Geometry check sheet. Reference: the model listing, model coordinates, mm. A direction names the side the tool comes from. Coordinates: 2 decimals unless noted, no trailing zeros. Write each loop counter-clockwise with the first axis right and the second up, starting at its lowest first coordinate (ties: lowest second). Pieces come first, ordered by that corner, then holes.
Autodesk Inventor part; units mm, degrees
ref_plane "YZ Plane" through (0, 0, 0) normal (1, 0, 0) x (0, 1, 0)
ref_plane "XZ Plane" through (0, 0, 0) normal (0, 1, 0) x (-1, 0, 0)
ref_plane "XY Plane" through (0, 0, 0) normal (0, 0, 1) x (1, 0, 0)
sketch "Sketch1" plane through (0, 0, 0) normal (0, 0, 1) x (1, 0, 0)
  line L0 (0, 0) -> (20, 0)
  line L1 (20, 0) -> (20, 3)
  line L2 (0, 3) -> (20, 3)
  line L3 (0, 0) -> (0, 3)
  line L4 (0, -95.4) -> (20, -95.4)
  line L5 (20, -95.4) -> (20, -92.4)
  line L6 (0, -92.4) -> (20, -92.4)
  line L7 (0, -95.4) -> (0, -92.4)
  line L8 (-7.5, 3) -> (0, 3) construction
  line L9 (20, 3) -> (27.5, 3) construction
  line L10 (20, -95.4) -> (27.5, -95.4) construction
  line L11 (-7.5, -95.4) -> (0, -95.4) construction
  line L12 (-7.5, 3) -> (27.5, 3)
  line L13 (27.5, -95.4) -> (-7.5, -95.4)
  line L14 (-7.5, 3) -> (27.5, -95.4) construction
  line L15 (27.5, 3) -> (-7.5, -95.4) construction
  line L16 (-7.5, -95.4) -> (-7.5, -70.567)
  line L17 (-7.5, -21.833) -> (-7.5, 3)
  line L18 (27.5, 3) -> (27.5, -21.833)
  line L19 (27.5, -70.567) -> (27.5, -95.4)
  arc A0 (27.5, -70.567) -> (27.5, -21.833) centre (10, -46.2) ccw
  arc A1 (-7.5, -21.833) -> (-7.5, -70.567) centre (10, -46.2) ccw
  dimension "d1" = 35
  dimension "d2" = 35
extrude "Extrusion1" add sketch "Sketch1" against normal blind 3 contours L0 L1 L12 L18 A0 L19 L13 L5 L6 L7 L16 A1 L17 L3
sketch "Sketch2" plane through (0, 0, -3) normal (0, 0, -1) x (-1, 0, 0)
  arc A0 (0.6, -86.2) -> (4.4, -86.2) centre (2.5, -86.2) ccw construction
  line L0 (0.6, -86.2) -> (0.6, -83.5) construction
  arc A1 (4.4, -83.5) -> (0.6, -83.5) centre (2.5, -83.5) ccw construction
  line L1 (4.4, -83.5) -> (4.4, -86.2) construction
  arc A2 (-1.5, -77.8) -> (-2.5, -78.8) centre (-1.5, -78.8) ccw construction
  line L2 (-2.5, -78.8) -> (-2.5, -91.4) construction
  line L3 (-2.5, -91.4) -> (7.5, -91.4) construction
  line L4 (7.5, -91.4) -> (7.5, -78.8) construction
  arc A3 (7.5, -78.8) -> (6.5, -77.8) centre (6.5, -78.8) ccw construction
  line L5 (6.5, -77.8) -> (-1.5, -77.8) construction
  arc A4 (-24.4, -86.2) -> (-20.6, -86.2) centre (-22.5, -86.2) ccw construction
  line L6 (-24.4, -86.2) -> (-24.4, -83.5) construction
  arc A5 (-20.6, -83.5) -> (-24.4, -83.5) centre (-22.5, -83.5) ccw construction
  line L7 (-20.6, -83.5) -> (-20.6, -86.2) construction
  arc A6 (-26.5, -77.8) -> (-27.5, -78.8) centre (-26.5, -78.8) ccw construction
  line L8 (-27.5, -78.8) -> (-27.5, -91.4) construction
  line L9 (-27.5, -91.4) -> (-17.5, -91.4) construction
  line L10 (-17.5, -91.4) -> (-17.5, -78.8) construction
  arc A7 (-17.5, -78.8) -> (-18.5, -77.8) centre (-18.5, -78.8) ccw construction
  line L11 (-18.5, -77.8) -> (-26.5, -77.8) construction
  arc A8 (4.4, -6.2) -> (0.6, -6.2) centre (2.5, -6.2) ccw construction
  line L12 (4.4, -6.2) -> (4.4, -8.9) construction
  arc A9 (0.6, -8.9) -> (4.4, -8.9) centre (2.5, -8.9) ccw construction
  line L13 (0.6, -8.9) -> (0.6, -6.2) construction
  arc A10 (6.5, -14.6) -> (7.5, -13.6) centre (6.5, -13.6) ccw construction
  line L14 (7.5, -13.6) -> (7.5, -1) construction
  line L15 (7.5, -1) -> (-2.5, -1) construction
  line L16 (-2.5, -1) -> (-2.5, -13.6) construction
  arc A11 (-2.5, -13.6) -> (-1.5, -14.6) centre (-1.5, -13.6) ccw construction
  line L17 (-1.5, -14.6) -> (6.5, -14.6) construction
  arc A12 (-20.6, -6.2) -> (-24.4, -6.2) centre (-22.5, -6.2) ccw construction
  line L18 (-20.6, -6.2) -> (-20.6, -8.9) construction
  arc A13 (-24.4, -8.9) -> (-20.6, -8.9) centre (-22.5, -8.9) ccw construction
  line L19 (-24.4, -8.9) -> (-24.4, -6.2) construction
  arc A14 (-18.5, -14.6) -> (-17.5, -13.6) centre (-18.5, -13.6) ccw construction
  line L20 (-17.5, -13.6) -> (-17.5, -1) construction
  line L21 (-17.5, -1) -> (-27.5, -1) construction
  line L22 (-27.5, -1) -> (-27.5, -13.6) construction
  arc A15 (-27.5, -13.6) -> (-26.5, -14.6) centre (-26.5, -13.6) ccw construction
  line L23 (-26.5, -14.6) -> (-18.5, -14.6) construction
  line L24 (-22.5, -86.2) -> (-22.5, -83.5) construction
  line L25 (2.5, -86.2) -> (2.5, -83.5) construction
  line L26 (2.5, -8.9) -> (2.5, -6.2) construction
  line L27 (-22.5, -8.9) -> (-22.5, -6.2) construction
  circle A16 centre (-22.5, -84.85) radius 1.9
  circle A17 centre (2.5, -84.85) radius 1.9
  circle A18 centre (2.5, -7.55) radius 1.9
  circle A19 centre (-22.5, -7.55) radius 1.9
  point P0 (0, 0)
extrude "Extrusion2" cut sketch "Sketch2" against normal blind 27.1625
sketch "Sketch3" plane through (0, 0, 0) normal (0, 0, 1) x (1, 0, 0)
  arc A0 (27.5, -70.567) -> (27.5, -21.833) centre (10, -46.2) ccw
  arc A1 (-7.5, -21.833) -> (-7.5, -70.567) centre (10, -46.2) ccw
  circle A2 centre (10, -46.2) radius 2
  point P0 (0, 0)
  dimension "d7" = 4
extrude "Extrusion3" cut sketch "Sketch3" against normal blind 14.4625
properties part number "Camera raiser"
1. Sectioned sample at D-D, the plane x = 22.5. Record the boundary of the cut face in (y, z), and give its area (3 significant figures).
Computed values:
outline: (-95.4, -3) - (-86.75, -3) - (-86.75, 0) - (-95.4, 0) - close; (-82.95, -3) - (-9.45, -3) - (-9.45, 0) - (-82.95, 0) - close; (-5.65, -3) - (3, -3) - (3, 0) - (-5.65, 0) - close
area: 272 mm2
2. Sectioned sample at C-C, the plane z = -2.55. Record the boundary of the cut face in (x, y).
Computed values:
outline: (-7.5, -95.4) - (0, -95.4) - (0, -92.4) - (20, -92.4) - (20, -95.4) - (27.5, -95.4) - (27.5, -70.57) arc R30 ccw to (27.5, -21.83) - (27.5, 3) - (20, 3) - (20, 0) - (0, 0) - (0, 3) - (-7.5, 3) - (-7.5, -21.83) arc R30 ccw to (-7.5, -70.57) - close; hole circle Ø3.8 at (-2.5, -84.85); hole circle Ø3.8 at (-2.5, -7.55); hole circle Ø4 at (10, -46.2); hole circle Ø3.8 at (22.5, -84.85); hole circle Ø3.8 at (22.5, -7.55)
3. Sectioned sample at B-B, the plane y = -84.85. Record the boundary of the cut face in (x, z).
Computed values:
outline: (-7.5, -3) - (-4.4, -3) - (-4.4, 0) - (-7.5, 0) - close; (-0.6, -3) - (20.6, -3) - (20.6, 0) - (-0.6, 0) - close; (24.4, -3) - (27.5, -3) - (27.5, 0) - (24.4, 0) - close
4. Gauge pin test, flat end, axial feed: pin 1 Ø0.9 at (y, z) = (2, -2) entering from +X. Record the tip position at first contact, or that the pin passes through.
Computed values:
pin 1: stops at x = 27.5
5. Thickness scan on line 1 along X through (y, z) = (-84.85, -1.7); line 2 along Y through (x, z) = (-2.5, -0.8); line 3 along X through (y, z) = (-6.5, -2.7). Record the ranges inside material, lowest first.
Computed values:
line 1: x = -7.5 to -4.4, -0.6 to 20.6, 24.4 to 27.5
line 2: y = -95.4 to -86.75, -82.95 to -9.45, -5.65 to 3
line 3: x = -7.5 to -4.08, -0.92 to 20.92, 24.08 to 27.5
6. Sectioned sample at A-A, the plane x = 10. Record the boundary of the cut face in (y, z).
Computed values:
outline: (-92.4, -3) - (-48.2, -3) - (-48.2, 0) - (-92.4, 0) - close; (-44.2, -3) - (0, -3) - (0, 0) - (-44.2, 0) - close
7. Access from +Z, -Z, +X, -X, +Y, -Y to the whole of each face (thin tool, end or side, straight path). Record for faces 5 (the flat face through (27.5, -83, -1)), 6 (the flat face through (0, -94, -1)), 7 (the flat face through (10, 0, -1)).
Computed values:
face 5: +Z, -Z, +X, -Y
face 6: +Z, -Z, -Y
face 7: +Z, -Z, +Y
8. Draft check along X on faces 1 (the flat face through (16, -46, -3)), 2 (the cylindrical face through (-20, -46, -1)), 3 (the cylindrical face through (-2.253, -5.666, -1.521)), 4 (the flat face through (27.5, -9, -1)). Enter one of: released by +X, released by -X, zero draft, split by the parting line, or undercut.
Computed values:
face 1: zero draft
face 2: released by -X
face 3: undercut
face 4: released by +X
